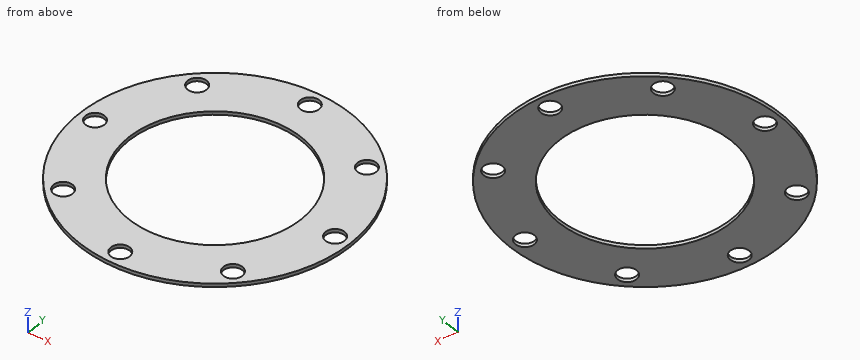
Autodesk Inventor part; units mm, degrees
ref_plane "YZ Plane" through (0, 0, 0) normal (1, 0, 0) x (0, 1, 0)
ref_plane "XZ Plane" through (0, 0, 0) normal (0, 1, 0) x (-1, 0, 0)
ref_plane "XY Plane" through (0, 0, 0) normal (0, 0, 1) x (1, 0, 0)
sketch "Sketch1" plane through (0, 0, 0) normal (0, 0, 1) x (1, 0, 0)
  circle A0 centre (0, 0) radius 100
  circle A1 centre (0, 0) radius 157.5
  dimension "d22" = 200
  dimension "d23" = 315
extrude "Plate1" add sketch "Sketch1" along normal blind 4
sketch "Sketch5" plane through (0, 0, 4) normal (0, 0, 1) x (1, 0, 0)
  circle A0 centre (0, 140) radius 11
  circle A1 centre (0, 0) radius 140 construction
  dimension "d25" = 280
  dimension "d24" = 22
extrude "Cut1" cut sketch "Sketch5" against normal blind 4
pattern_circular "Circular Pattern1" count 8 over 360 about axis through (0, 0, 0) along (0, 0, 1) of "Cut1"
equation "\"d26\" = Thickness"
equation "\"d2\" = Thickness"
equation "\"BendReliefWidth\" = Thickness"
equation "\"BendReliefDepth\" = 0.5 * Thickness"
equation "\"CornerReliefSize\" = 4 * Thickness"
equation "\"MinimumRemnant\" = 2 * Thickness"
equation "\"TransitionRadius\" = BendRadius"
equation "\"JacobiRadiusSize\" = BendRadius"
equation "\"GapSize\" = Thickness"
properties part number "ANP 1411 BOTTOM DS main flange" material "Stainless Steel"
Can you work these out from the model? Positions are in its coordinate system, mm. Coordinates: 2 decimals unless noted, no trailing zeros. Write each loop counter-clockwise with the first axis right and the second up, starting at its lowest first coordinate (ties: lowest second). Pieces come first, ordered by that corner, then holes.
Q1. Imagine slicing it at A-A, the plane x = 0. List the corners of the cut face in (y, z) for me.
Results found:
outline: (-157.5, 0) - (-151, 0) - (-151, 4) - (-157.5, 4) - close; (-129, 0) - (-100, 0) - (-100, 4) - (-129, 4) - close; (100, 0) - (129, 0) - (129, 4) - (100, 4) - close; (151, 0) - (157.5, 0) - (157.5, 4) - (151, 4) - close
Q2. Imagine slicing it at B-B, the plane y = 140. List the corners of the cut face in (x, z) for me, plus the area to 3 significant figures.
Results found:
outline: (-72.15, 0) - (-11, 0) - (-11, 4) - (-72.15, 4) - close; (11, 0) - (72.15, 0) - (72.15, 4) - (11, 4) - close
area: 489 mm2
Q3. For P1, Ø17.5, axis at x = 98.99, y = 98.99, coming from the +Z side; P2, Ø1, axis at y = -81, z = 3.5, coming from the +X side, each with a flat end and sliding along its axis, tell me the tip position at first contact or that it passes through.
Results found:
P1: passes through
P2: stops at x = 135.37
Q4. Please list where these lines run through material, in increasing order: L1, parallel to Y at x = 0, z = 1.9; L2, parallel to Y at x = -2, z = 3.85; L3, parallel to X at y = 103.5, z = 2.
Results found:
L1: y = -157.5 to -151, -129 to -100, 100 to 129, 151 to 157.5
L2: y = -157.49 to -150.82, -129.18 to -99.98, 99.98 to 129.18, 150.82 to 157.49
L3: x = -118.72 to -109.03, -88.96 to 88.96, 109.03 to 118.72
Q5. Imagine slicing it at D-D, the plane x = -58. List the corners of the cut face in (y, z) for me.
Results found:
outline: (-146.43, 0) - (-81.46, 0) - (-81.46, 4) - (-146.43, 4) - close; (81.46, 0) - (146.43, 0) - (146.43, 4) - (81.46, 4) - close
